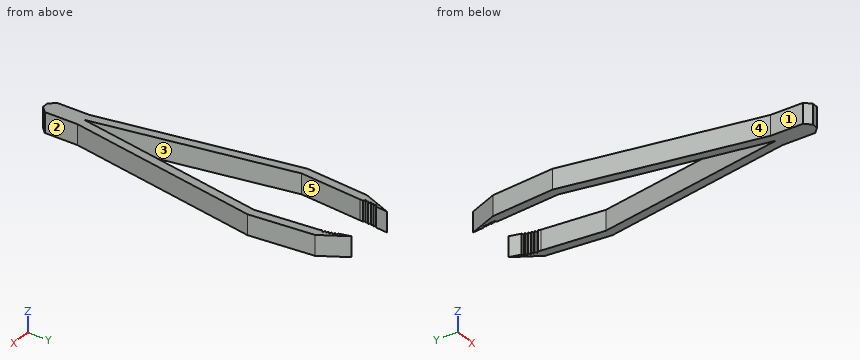
```python
from build123d import *

# Parameters (mm, degrees)
F0_W     = 6
F0_H     = 13.295454
F1_DEPTH = 7
F2_SIZE  = 2


with BuildPart() as f1:
    # F0 (on Top) → F1 (new body)
    with BuildSketch(Plane.XY):
        Polygon((-8.782924, 66.457867), (-12.721482, 56.78893), (-9.735013, 56.503294), (-9.639804, 57.498751), (-10.454291, 58.078933), (-9.544595, 58.494208), (-10.359082, 59.07439), (-9.449386, 59.489666), (-10.263873, 60.069848), (-9.354177, 60.485123), (-10.168664, 61.065305), (-9.258968, 61.48058), (-10.073455, 62.060762), (-9.16376, 62.476038), align=None)
        Polygon((-14.638909, 34.872646), (-2.830833, -32.094281), (3.169167, -32.094281), (14.977244, 34.872646), (13.059817, 56.78893), (10.112168, 56.059576), (11.954237, 35.004634), (0.169167, -31.831815), (-11.615902, 35.004634), (-9.735013, 56.503294), (-12.721482, 56.78893), align=None)
        with Locations((0.169167, -38.742008)):
            Rectangle(F0_W, F0_H)
        Polygon((10.112168, 56.059576), (13.059817, 56.78893), (7.710246, 65.766829), (8.671014, 61.883928), (9.631783, 61.606578), (8.911207, 60.913202), (9.871976, 60.635852), (9.151399, 59.942477), (10.112168, 59.665127), (9.391591, 58.971752), (10.35236, 58.694402), (9.631783, 58.001026), (10.592552, 57.723676), (9.871976, 57.030301), align=None)
    extrude(amount=F1_DEPTH)

    # F2
    f2_edges = [f1.edges().sort_by_distance(p)[0] for p in [
        (-2.830833, -45.389735, 3.5),
        (3.169167, -45.389735, 3.5),
    ]]
    chamfer(f2_edges, length=F2_SIZE)


solid = f1.part
```
Read the model definition and answer for the solid it produces. Units are mm, in the model's axes. Face numbers are marked on the shaded views. A direction names the side the tool comes from. Coordinates: 2 decimals unless noted, no trailing zeros. Write each loop counter-clockwise with the first axis right and the second up, starting at its lowest first coordinate (ties: lowest second). Pieces come first, ordered by that corner, then holes. Notation, with made-up numbers: (89, 72.25) -> (95, 72.25) arc R13 cw to (95, 97.25) -> close; hole circle Ø6 at (-25, 64.25). An arc over 180 degrees is marked (long way). Write item = value, one per line.
(1) Straight lines are drawn through the part: L1, parallel to X at y = -38.5, z = 2.5; L2, parallel to X at y = 28, z = 5; L3, parallel to X at y = -28, z = 6.25. For each, find the intervals that lie inside material, in ascending order. Write a range as from..to.
From the geometry:
L1 = -2.83..3.17
L2 = -13.43..-10.38, 10.72..13.77
L3 = -3.55..-0.51, 0.84..3.89
(2) Section B-B on y = -37.5 is taken. Write down the section's boundary in (x, z).
From the geometry:
outline = (-2.83, 0) -> (3.17, 0) -> (3.17, 7) -> (-2.83, 7) -> close
(3) Which of the six approach directions +Z, -Z, +X, -X, +Y, -Y give full straight-line access (tool end or side, diameter ignored) to the marked faces 4 and 5?
From the geometry:
face_4 = +Z, -Z, -X, -Y
face_5 = +Z, -Z
(4) Section A-A on y = 29 is taken. Write down the section's boundary in (x, z), plus the area to 3 significant figures.
From the geometry:
outline = (-13.6, 0) -> (-10.56, 0) -> (-10.56, 7) -> (-13.6, 7) -> close; (10.9, 0) -> (13.94, 0) -> (13.94, 7) -> (10.9, 7) -> close
area = 42.6 mm2
(5) For a pull along X with two mould halves and no side action, classify the marked faces 1, 2 and 3 as +X half, -X half, draft (parallel to the pull), parting line (faces both ways), or undercut.
From the geometry:
face_1 = -X half
face_2 = +X half
face_3 = undercut
(6) Given pin 1 Ø3 at (y, z) = (-14, 5.5) entering from +X, flat-ended and moving along its own axis, determine where the tip first touches the part or whether it passes through.
From the geometry:
pin_1 = 6.62
(7) Section C-C on x = 6.75 is taken. Write down the section's boundary in (y, z).
From the geometry:
outline = (-11.79, 0) -> (5.49, 0) -> (5.49, 7) -> (-11.79, 7) -> close
